```python
from build123d import *

# Parameters (mm, degrees)
SKETCH1_W           = 12.4
SKETCH1_H           = 13.2
BOSS_EXTRUDE1_DEPTH = 5
FILLET1_R           = 2
SKETCH2_R           = 3.4
BOSS_EXTRUDE2_DEPTH = 5
SKETCH3_R           = 3
BOSS_EXTRUDE3_DEPTH = 10
CHAMFER1_SIZE       = 1.5
CHAMFER1_SIZE2      = 0.699461487
SKETCH4_R           = 0.5
CUT_EXTRUDE1_DEPTH  = 18.521415468
SKETCH5_W           = 6.05122926
SKETCH5_H           = 1.5
CUT_EXTRUDE2_DEPTH  = 7


with BuildPart() as part:
    # Sketch1 → Boss-Extrude1 (new body)
    with BuildSketch(Plane(origin=(0, 0, 0), x_dir=(1, 0, 0), z_dir=(0, 1, 0))):
        Rectangle(SKETCH1_W, SKETCH1_H)
    extrude(amount=BOSS_EXTRUDE1_DEPTH)

    # Fillet1
    fillet1_edges = [part.edges().sort_by_distance(p)[0] for p in [
        (-6.2, 2.5, -6.6),
        (6.2, 2.5, -6.6),
        (6.2, 2.5, 6.6),
        (-6.2, 2.5, 6.6),
    ]]
    fillet(fillet1_edges, radius=FILLET1_R)

    # Sketch2 → Boss-Extrude2 (add)
    with BuildSketch(Plane(origin=(0, 5, 0), x_dir=(1, 0, 0), z_dir=(0, 1, 0))):
        with Locations(Location((0, 0, 0), (0, 0, 270))):
            Circle(SKETCH2_R)
    extrude(amount=BOSS_EXTRUDE2_DEPTH)

    # Sketch3 → Boss-Extrude3 (add)
    with BuildSketch(Plane(origin=(0, 10, 0), x_dir=(1, 0, 0), z_dir=(0, 1, 0))):
        with Locations(Location((0, 0, 0), (0, 0, 270))):
            Circle(SKETCH3_R)
    extrude(amount=BOSS_EXTRUDE3_DEPTH)

    # Chamfer1
    chamfer1_edges = [part.edges().sort_by_distance(p)[0] for p in [
        (0, 20, -3),
    ]]
    chamfer1_side = [part.faces().sort_by_distance(p)[0] for p in [
        (0, 15, -3),
    ]]
    chamfer(chamfer1_edges, length=CHAMFER1_SIZE, length2=CHAMFER1_SIZE2, reference=chamfer1_side[0])

    # Sketch4 → Cut-Extrude1 (cut, through all)
    with BuildSketch(Plane(origin=(0, 5, 0), x_dir=(1, 0, 0), z_dir=(0, 1, 0))):
        with Locations(Location((4.1, -5.1, 0), (0, 0, 270))):
            Circle(SKETCH4_R)
        with Locations(Location((-4.1, -5.1, 0), (0, 0, 270))):
            Circle(SKETCH4_R)
        with Locations(Location((-4.1, 5.1, 0), (0, 0, 270))):
            Circle(SKETCH4_R)
        with Locations(Location((4.1, 5.1, 0), (0, 0, 270))):
            Circle(SKETCH4_R)
    extrude(amount=-CUT_EXTRUDE1_DEPTH, mode=Mode.SUBTRACT)

    # Sketch5 → Cut-Extrude2 (cut)
    with BuildSketch(Plane(origin=(0, 20, 0), x_dir=(1, 0, 0), z_dir=(0, 1, 0))):
        with Locations((0.02561463, 2.25)):
            Rectangle(SKETCH5_W, SKETCH5_H)
    extrude(amount=-CUT_EXTRUDE2_DEPTH, mode=Mode.SUBTRACT)


solid = part.part
```
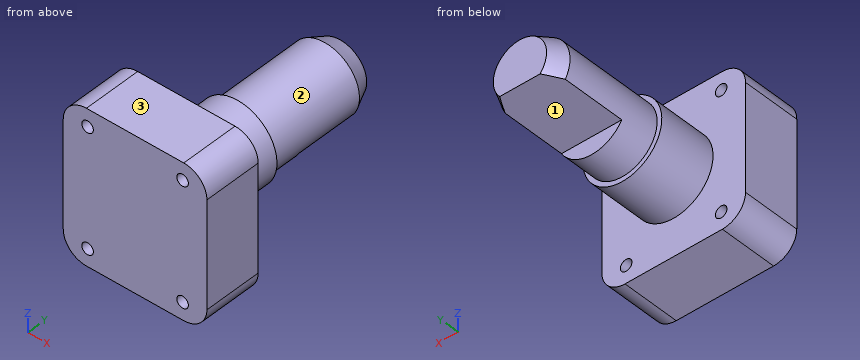
The model under review builds one solid part; all positions refer to its coordinate system, in mm. Face numbers are marked on the shaded views. A direction names the side the tool comes from. Round coordinates to 2 decimals unless told otherwise and drop trailing zeros. Order: outer loops, then holes, each group sorted by start corner. A loop starts at its lowest first (then second) coordinate and runs counter-clockwise, first axis right, second up.
(1) Take a section at D-D, the plane z = 0. State the section outline as (x, y) points, plus the area to 3 significant figures.
Working result:
outline: (-6.2, 0) - (6.2, 0) - (6.2, 5) - (3.4, 5) - (3.4, 10) - (3, 10) - (3, 18.5) - (2.3, 20) - (-2.3, 20) - (-3, 18.5) - (-3, 10) - (-3.4, 10) - (-3.4, 5) - (-6.2, 5) - close
area: 155 mm2
(2) For P1, Ø0.8, axis at x = -1, z = -2.5, coming from the +Y side; P2, Ø4, axis at x = 1, y = 18, coming from the -Z side, all flat-tipped, find the tip position at first contact; note any pin that passes through.
Working result:
P1: stops at y = 13
P2: stops at z = -1.5
(3) Tool access review of the marked faces 1, 2 and 3: name each direction out of +Z, -Z, +X, -X, +Y, -Y from which nothing blocks a thin tool from reaching the whole face with its end or side.
Working result:
face 1: -Z, +X, -X, +Y
face 2: +Y
face 3: +Z, +X, -X, +Y, -Y
(4) Wall thickness on L1, parallel to X at y = 1, z = -5.1; L2, parallel to Y at x = 2, z = 5; L3, parallel to Y at x = 0.75, z = -1.75: over which ranges is each line inside the solid? List them lowest first.
Working result:
L1: x = -6.14 to -4.6, -3.6 to 3.6, 4.6 to 6.14
L2: y = 0 to 5
L3: y = 0 to 13
(5) Take a section at A-A, the plane y = 2.75. State the section outline as (x, z) points.
Working result:
outline: (-6.2, -4.6) arc R2 ccw to (-4.2, -6.6) - (4.2, -6.6) arc R2 ccw to (6.2, -4.6) - (6.2, 4.6) arc R2 ccw to (4.2, 6.6) - (-4.2, 6.6) arc R2 ccw to (-6.2, 4.6) - close; hole circle Ø1 at (-4.1, -5.1); hole circle Ø1 at (-4.1, 5.1); hole circle Ø1 at (4.1, -5.1); hole circle Ø1 at (4.1, 5.1)
(6) Take a section at B-B, the plane x = 0. State the section outline as (y, z) points.
Working result:
outline: (0, -6.6) - (5, -6.6) - (5, -3.4) - (10, -3.4) - (10, -3) - (13, -3) - (13, -1.5) - (20, -1.5) - (20, 2.3) - (18.5, 3) - (10, 3) - (10, 3.4) - (5, 3.4) - (5, 6.6) - (0, 6.6) - close
(7) Take a section at C-C, the plane z = -5.1. State the section outline as (x, y) points.
Working result:
outline: (-6.14, 0) - (-4.6, 0) - (-4.6, 5) - (-6.14, 5) - close; (-3.6, 0) - (3.6, 0) - (3.6, 5) - (-3.6, 5) - close; (4.6, 0) - (6.14, 0) - (6.14, 5) - (4.6, 5) - close
